```python
from build123d import *


with BuildPart() as part:
    # Sketch2 → Revolve1 (revolve)
    with BuildSketch(Plane(origin=(0, 0, 0), x_dir=(0, 0, -1), z_dir=(1, 0, 0))):
        with BuildLine():
            Line((-11.5, 28), (-11.5, 20))
            Line((-11.5, 20), (-9.5, 20))
            Line((-9.5, 20), (-9.5, 30))
            Line((-9.5, 30), (-10.547037499, 30))
            ThreePointArc((-10.547037499, 30), (-12.849730042, 29.088218197), (-15.074481749, 28))
            Line((-15.074481749, 28), (-11.5, 28))
        make_face()
        with BuildLine():
            ThreePointArc((-15.570484899, 30), (-21.985230431, 25.672741243), (-27.247752201, 20))
            Line((-27.247752201, 20), (-24.723268392, 20))
            ThreePointArc((-24.723268392, 20), (-20.296926592, 24.480089275), (-15.074481749, 28))
            ThreePointArc((-15.074481749, 28), (-12.849730042, 29.088218197), (-10.547037499, 30))
            Line((-10.547037499, 30), (-15.570484899, 30))
        make_face()
    revolve(axis=Axis((0, 0, 0), (0, 1, 0)))


solid = part.part
```
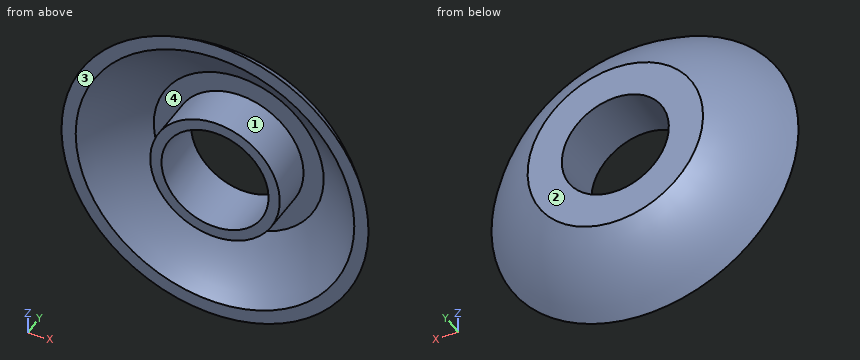
Build history of the part. All positions in model axes, mm. Face numbers are marked on the shaded views. A direction names the side the tool comes from. Give positions to 0.01 mm unless a question says otherwise; leave off trailing zeros. Loops run counter-clockwise (first coordinate to the right, second up) from the corner with the lowest first, then second, coordinate; pieces in that order, holes last. Notation, with made-up numbers: (-12, -2.5) - (-7, -2.5) arc R28 cw to (-7, 32.5) - close; hole circle Ø5 at (27.25, 24). An arc over 180 degrees is marked (long way). Use a Markdown table: item, result.
(1) Pull direction X, two halves, no side cores. Call the marked faces 1 and 2: +X half, -X half, draft (parallel to the pull), parting line (faces both ways), or undercut.
Taken from the geometry:
| item | result |
|---|---|
| face 1 | undercut |
| face 2 | draft |
(2) Band-saw the part on D-D (x = 14). Give the cut face in (y, z), and give its area (3 significant figures).
Taken from the geometry:
| item | result |
|---|---|
| outline | (20, -23.38) arc R30.76 ccw to (30, -6.81) - (30, 6.81) arc R30.76 ccw to (20, 23.38) - (20, 20.38) arc R28.55 cw to (28, 5.59) - (28, -5.59) arc R28.55 cw to (20, -20.38) - close |
| area | 106 mm2 |
(3) Band-saw the part on A-A (z = 0). Give the cut face in (x, y).
Taken from the geometry:
| item | result |
|---|---|
| outline | (-27.25, 20) - (-24.72, 20) arc R31.8 cw to (-15.07, 28) - (-11.5, 28) - (-11.5, 20) - (-9.5, 20) - (-9.5, 30) - (-15.57, 30) arc R33.8 ccw to start; (9.5, 20) - (11.5, 20) - (11.5, 28) - (15.07, 28) arc R31.8 cw to (24.72, 20) - (27.25, 20) arc R33.8 ccw to (15.57, 30) - (9.5, 30) - close |
(4) Band-saw the part on B-B (x = 0). Give the cut face in (y, z).
Taken from the geometry:
| item | result |
|---|---|
| outline | (20, -27.25) arc R33.8 ccw to (30, -15.57) - (30, -9.5) - (20, -9.5) - (20, -11.5) - (28, -11.5) - (28, -15.07) arc R31.8 cw to (20, -24.72) - close; (20, 9.5) - (30, 9.5) - (30, 15.57) arc R33.8 ccw to (20, 27.25) - (20, 24.72) arc R31.8 cw to (28, 15.07) - (28, 11.5) - (20, 11.5) - close |
(5) Band-saw the part on C-C (y = 21.25). Give the cut face in (x, z) (1 decimal).
Taken from the geometry:
| item | result |
|---|---|
| outline | circle Ø52.6 at (0, 0); circle Ø23 at (0, 0); hole circle Ø47.3 at (0, 0); hole circle Ø19 at (0, 0) |
(6) Which spindle directions (+Z, -Z, +X, -X, +Y, -Y) get a long thin tool onto all of the face, cutting with end or side? Do the marked faces 3 and 4. Say none if no direction does.
Taken from the geometry:
| item | result |
|---|---|
| face 3 | +Z, -Z, +X, -X, -Y |
| face 4 | -Y |
(7) Drop flat-ended pins along their axis: pin 1 Ø5 at (x, y) = (14, 28.5) entering from +Z; pin 2 Ø2 at (x, y) = (18.5, 26) entering from -Z; pin 3 Ø4 at (x, z) = (-21.5, -6) entering from -Y. Give the stop position or say it passes through.
Taken from the geometry:
| item | result |
|---|---|
| pin 1 | z = 16.93 |
| pin 2 | z = -13.68 |
| pin 3 | y = 20.49 |
(8) Wall check: line 1 along X through (y, z) = (26.75, 0); line 2 along X through (y, z) = (25.5, -1.5); line 3 along Z through (x, y) = (-8, 23.25). Give the ranges that are in metal, low to high.
Taken from the geometry:
| item | result |
|---|---|
| line 1 | -20.66 to -17.2, -11.5 to -9.5, 9.5 to 11.5, 17.2 to 20.66 |
| line 2 | -22.13 to -18.94, -11.4 to -9.38, 9.38 to 11.4, 18.94 to 22.13 |
| line 3 | -23.19 to -20.17, -8.26 to -5.12, 5.12 to 8.26, 20.17 to 23.19 |
